The model under review builds one solid part; all positions refer to its coordinate system, in mm. Face numbers are marked on the shaded views. A direction names the side the tool comes from. Round coordinates to 2 decimals unless told otherwise and drop trailing zeros. Loops run counter-clockwise (first coordinate to the right, second up) from the corner with the lowest first, then second, coordinate; pieces in that order, holes last. Notation, with made-up numbers: M 73.25,20 L 103.25,20 A26 ccw 103.25,56 Z; hole C 48,0.25 d1. An arc over 180 degrees is marked long. Answer in a Markdown table with one row per item. Add a question column.
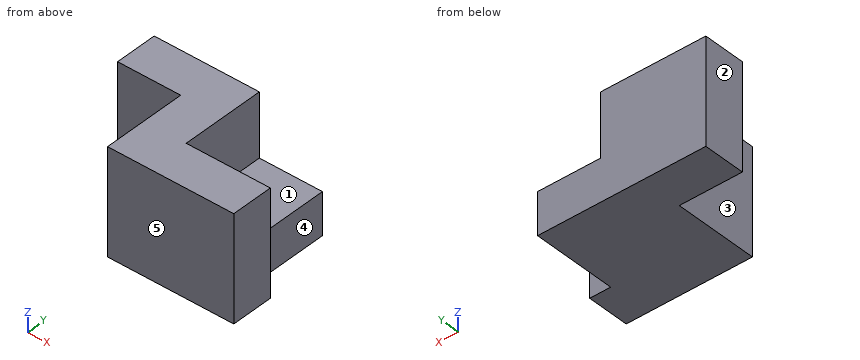
from build123d import *

# Parameters (mm, degrees)
CROQUIS2_W              = 90
CROQUIS2_H              = 60
SALIENTE_EXTRUIR1_DEPTH = 50
CROQUIS3_W              = 50
CROQUIS3_H              = 40
CORTAR_EXTRUIR3_DEPTH   = 30
CROQUIS5_W              = 30
CROQUIS5_H              = 30
CORTAR_EXTRUIR4_DEPTH   = 40


with BuildPart() as part:
    # Croquis2 → Saliente-Extruir1 (new body)
    with BuildSketch(Plane.XY):
        Rectangle(CROQUIS2_W, CROQUIS2_H)
    extrude(amount=SALIENTE_EXTRUIR1_DEPTH)

    # Croquis3 → Cortar-Extruir3 (cut)
    with BuildSketch(Plane.ZY.offset(45)):
        with Locations((25, -10)):
            Rectangle(CROQUIS3_W, CROQUIS3_H)
    extrude(amount=-CORTAR_EXTRUIR3_DEPTH, mode=Mode.SUBTRACT)

    # Croquis5 → Cortar-Extruir4 (cut)
    with BuildSketch(Plane(origin=(0, 30, 0), x_dir=(1, 0, 0), z_dir=(0, 1, 0))):
        with Locations((20, -35)):
            Rectangle(CROQUIS5_W, CROQUIS5_H)
        Polygon((45, -50), (45, 0), (35, 0), (35, -20), (35, -50), align=None)
    extrude(amount=-CORTAR_EXTRUIR4_DEPTH, mode=Mode.SUBTRACT)


solid = part.part
1. To check wall thickness, follow probe 1 along X at (y, z) = (20, 45.5); probe 2 along Y at (x, z) = (-37, 13); probe 3 along X at (y, z) = (13, 18). State the ranges of each line that lie inside material, in increasing order.
2. Take a section at B-B, the plane y = 12.5. State the section outline as (x, z) points.
3. Take a section at C-C, the plane x = 17. State the section outline as (y, z) points.
4. Take a section at A-A, the plane z = 35.5. State the section outline as (x, y) points.
5. Machinability: for the marked faces 1, 2, 3, 4 and 5, which of the approach directions +Z, -Z, +X, -X, +Y, -Y give a long, thin tool a straight path to every point of the face, cutting with its end or side? Answer none if there is none.
6. Take a section at D-D, the plane z = 9. State the section outline as (x, y) points.
7. For pin 1 Ø9 at (x, y) = (23.5, 19) entering from +Z; pin 2 Ø8 at (y, z) = (-5.5, 22.5) entering from +X; pin 3 Ø24 at (x, z) = (-32.5, 16.5) entering from -Y, all flat-tipped, find the tip position at first contact; note any pin that passes through.
Check sheet entries:
| question | item | result |
|---|---|---|
| 1 | probe 1 | x = -45 to 5 |
| 1 | probe 2 | y = 10 to 30 |
| 1 | probe 3 | x = -45 to 35 |
| 2 | outline | M -45,0 L 35,0 L 35,20 L 5,20 L 5,50 L -45,50 Z |
| 3 | outline | M -30,0 L 30,0 L 30,20 L -10,20 L -10,50 L -30,50 Z |
| 4 | outline | M -45,10 L -15,10 L -15,-30 L 45,-30 L 45,-10 L 5,-10 L 5,30 L -45,30 Z |
| 5 | face 1 | +Z, +X, +Y |
| 5 | face 2 | +Z, -Z, -X, +Y, -Y |
| 5 | face 3 | +Z, -Z, -X, -Y |
| 5 | face 4 | +Z, -Z, +X, +Y |
| 5 | face 5 | +Z, -Z, +X, -X, -Y |
| 6 | outline | M -45,10 L -15,10 L -15,-30 L 45,-30 L 45,-10 L 35,-10 L 35,30 L -45,30 Z |
| 7 | pin 1 | stops at z = 20 |
| 7 | pin 2 | stops at x = 35 |
| 7 | pin 3 | stops at y = 10 |
